The listing builds one solid part. Answer for the finished solid, in the listing's coordinates (mm). A direction names the side the tool comes from. Give positions to 0.01 mm unless a question says otherwise; leave off trailing zeros. Loops run counter-clockwise (first coordinate to the right, second up) from the corner with the lowest first, then second, coordinate; pieces in that order, holes last. Notation, with made-up numbers: M -17.75,45.5 L -1.75,45.5 A16 cw -1.75,72.5 Z; hole C 78.5,66 d8. An arc over 180 degrees is marked long. One line per item, written item: value. Start each with the question number.
Q1. A cutting plane is placed at C-C, the plane z = 3.5. Determine the outline of the cut face in (x, y).
Q2. Flat-ended cylindrical pins translate along their axes: pin 1 (1 mm diameter, centred on x = -8.5, y = 6.5, fed in from +Z); pin 2 (1.1 mm diameter, centred on x = 12, z = 6.5, fed in from -Y); pin 3 (1.5 mm diameter, centred on x = -3.5, z = 4.5, fed in from -Y). Find the tip coordinate at first contact, or state that the pin passes through.
Q3. A cutting plane is placed at B-B, the plane x = 11. Determine the outline of the cut face in (y, z).
Q4. A cutting plane is placed at D-D, the plane y = 20.5. Determine the outline of the cut face in (x, z).
Q5. A cutting plane is placed at A-A, the plane z = 6.75. Determine the outline of the cut face in (x, y), and give its area (3 significant figures).
Q6. Consider L1, parallel to X at y = 7.75, z = 4; L2, parallel to Y at x = -11.5, z = 2; L3, parallel to X at y = 8.5, z = 2. Determine where each line is inside the solid, lowest interval first.
Q7. For faces 1 (the flat face through (12, 18.5, 7)), 2 (the flat face through (-0.1, 24.5, 6.16)), 3 (the flat face through (-13, 12, 5)), 4 (the cylindrical face through (12.57, 9.12, 2.11)), 5 (the flat face through (-14, 13, 4)), determine the directions among +Z, -Z, +X, -X, +Y, -Y from which every point of the face is accessible in a straight line to the end or side of a thin tool.
from build123d import *

# Parameters (mm, degrees)
SKETCH_W     = 28
SKETCH_H     = 25
PAD_DEPTH    = 1.66
PAD001_DEPTH = 4.5
PAD002_DEPTH = 6.5
FILLET_R     = 1.5


with BuildPart() as part:
    # Sketch → Pad (new body)
    with BuildSketch(Plane.XY):
        with Locations((0, 12.5)):
            Rectangle(SKETCH_W, SKETCH_H)
    extrude(amount=PAD_DEPTH)

    # Sketch001 → Pad001 (new body)
    with BuildSketch(Plane.XY.offset(1.66)):
        Polygon((-14, 0), (-13, 0), (-13, 24), (13, 24), (13, 0), (14, 0), (14, 25), (-14, 25), align=None)
    extrude(amount=PAD001_DEPTH)

    # Sketch002 → Pad002 (new body)
    with BuildSketch(Plane(origin=(0, 25, 0), x_dir=(-1, 0, 0), z_dir=(0, 1, 0))):
        Polygon((-10.5, 6.16), (-10.5, 7.16), (-14, 7.16), (-14, 1.66), (-10.5, 1.66), (-10.5, 4.26), (-13, 4.26), (-13, 6.16), align=None)
    pad002 = extrude(amount=-PAD002_DEPTH)

    # Mirrored: Pad002 across Sketch002 V_Axis
    add(pad002.mirror(Plane(origin=(0, 25, 0), x_dir=(0, 1, 0), z_dir=(-1, 0, 0))))

    # Fillet
    fillet_edges = [part.edges().sort_by_distance(p)[0] for p in [
        (0, 24, 1.66),
        (13, 9.25, 1.66),
        (-13, 9.25, 1.66),
    ]]
    fillet(fillet_edges, radius=FILLET_R)


solid = part.part
Answer block:
1. outline: M -14,0 L -13,0 L -13,18.5 L -10.5,18.5 L -10.5,24 L 10.5,24 L 10.5,18.5 L 13,18.5 L 13,0 L 14,0 L 14,25 L -14,25 Z
2. pin 1: z = 1.66
2. pin 2: y = 18.5
2. pin 3: y = 24
3. outline: M 0,0 L 25,0 L 25,7.16 L 18.5,7.16 L 18.5,6.16 L 24,6.16 L 24,4.26 L 18.5,4.26 L 18.5,1.66 L 0,1.66 Z
4. outline: M -14,0 L 14,0 L 14,7.16 L 10.5,7.16 L 10.5,6.16 L 13,6.16 L 13,4.26 L 10.5,4.26 L 10.5,1.66 L -10.5,1.66 L -10.5,4.26 L -13,4.26 L -13,6.16 L -10.5,6.16 L -10.5,7.16 L -14,7.16 Z
5. outline: M -14,18.5 L -10.5,18.5 L -10.5,25 L -14,25 Z; M 10.5,18.5 L 14,18.5 L 14,25 L 10.5,25 Z
5. area: 45.5 mm^2
6. L1: -14 to -13, 13 to 14
6. L2: 18.5 to 25
6. L3: -14 to -12.45, 12.45 to 14
7. face 1: +Z, +X, -X, -Y
7. face 2: +Z, +Y, -Y
7. face 3: -Y
7. face 4: +Z, -Y
7. face 5: +Z, -Z, -X, +Y, -Y
